Geometry: see drawing. Coordinates: mm, zero at the bounding-box minimum. A direction names the side the tool comes from. Coordinates: 2 decimals unless noted, no trailing zeros. Loops run counter-clockwise (first coordinate to the right, second up) from the corner with the lowest first, then second, coordinate; pieces in that order, holes last. Notation, with made-up numbers: M 64,-12 L 116,-12 A20 cw 116,12 Z; hole C 78,83.5 d10. An arc over 180 degrees is marked long. One line per question, with ' | ' between items. Start each with the question number.
1. Section query C-C, the plane z = 35.5. Output: boundary loops of the cut face in (x, y), and give its area (3 significant figures).
2. Section query A-A, the plane z = 19.05. Output: boundary loops of the cut face in (x, y).
3. Section query B-B, the plane x = 88. Output: boundary loops of the cut face in (y, z).
4. Pin query (flat end, axial travel): P1, Ø2, axis at x = 141.5, y = 20.5, coming from the -Z side; P2, Ø8, axis at x = 104.5, z = 42, coming from the +Y side; P3, Ø2.5, axis at y = 28, z = 48.5, coming from the -X side. Return the tip coordinate at first contact, or that it passes through.
5. Ray query, probe 1 along X at (y, z) = (28, 19); probe 2 along Z at (x, y) = (170.5, 13); probe 3 along Y at (x, z) = (114, 74). Return the intervals inside material, ascending.
6. Access query for the marked faces 1, 2 and 3. Directions: +Z, -Z, +X, -X, +Y, -Y. A direction counts if a zero-diameter tool reaches every point of the face in a straight line with its end or side. Return the directions, or none.
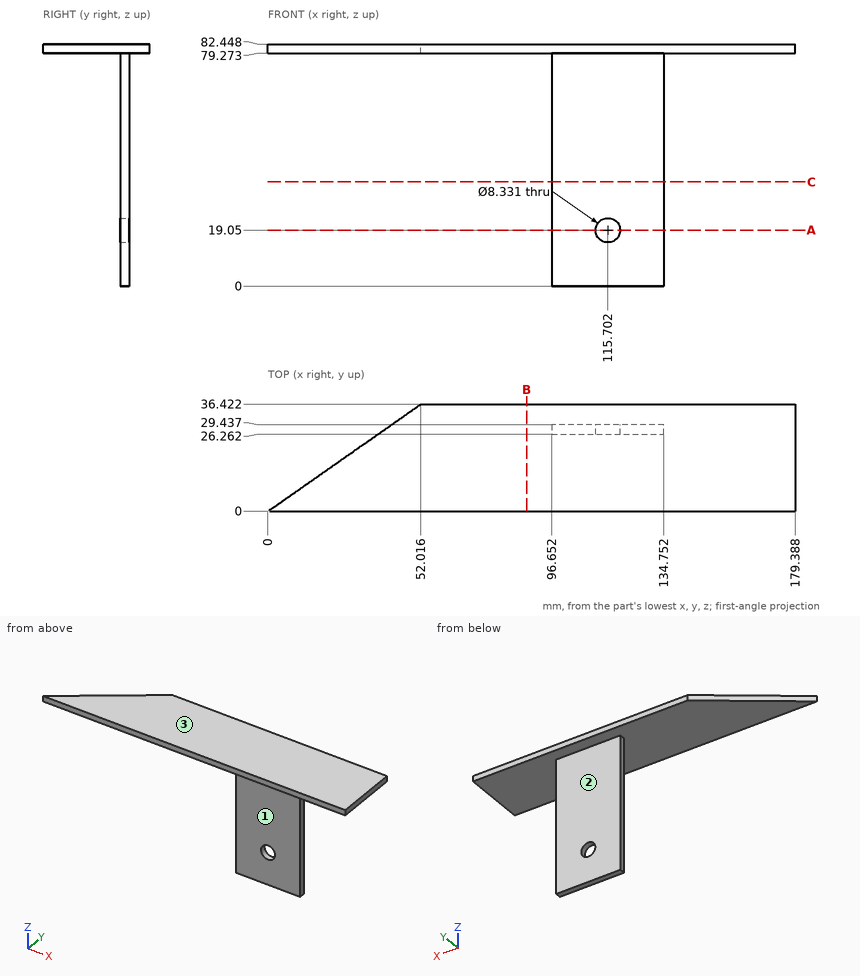
Taken from the geometry:
1) outline: M 96.65,26.26 L 134.75,26.26 L 134.75,29.44 L 96.65,29.44 Z | area: 121 mm^2
2) outline: M 96.65,26.26 L 111.54,26.26 L 111.54,29.44 L 96.65,29.44 Z; M 119.87,26.26 L 134.75,26.26 L 134.75,29.44 L 119.87,29.44 Z
3) outline: M 0,79.27 L 36.42,79.27 L 36.42,82.45 L 0,82.45 Z
4) P1: z = 79.27 | P2: y = 29.44 | P3: x = 96.65
5) probe 1: 96.65 to 111.54, 119.87 to 134.75 | probe 2: 79.27 to 82.45 | probe 3: 26.26 to 29.44
6) face 1: -Z, +X, -X, -Y | face 2: -Z, +X, -X, +Y | face 3: +Z, +X, -X, +Y, -Y
